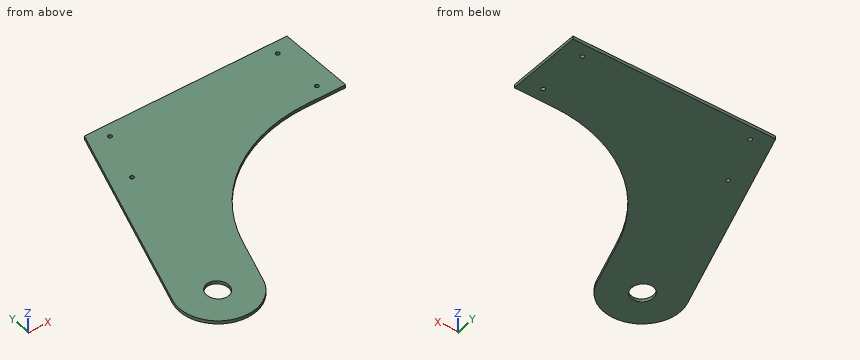
Autodesk Inventor part; units mm, degrees
ref_plane "YZ Plane" through (0, 0, 0) normal (1, 0, 0) x (0, 1, 0)
ref_plane "XZ Plane" through (0, 0, 0) normal (0, 1, 0) x (-1, 0, 0)
ref_plane "XY Plane" through (0, 0, 0) normal (0, 0, 1) x (1, 0, 0)
sketch "Sketch1" plane through (0, 0, 0) normal (0, 0, 1) x (1, 0, 0)
  arc A0 (219.754, -304.8) -> (225.7704, -296.4188) centre (219.754, -298.45) ccw
  line L0 (225.7704, -296.4188) -> (30.0819, 283.206)
  arc A1 (30.0819, 283.206) -> (-30.0819, 283.206) centre (0, 273.05) ccw
  line L1 (-30.0819, 283.206) -> (-225.7704, -296.4188)
  arc A2 (-225.7704, -296.4188) -> (-219.754, -304.8) centre (-219.754, -298.45) ccw
  line L2 (-219.754, -304.8) -> (219.754, -304.8)
  line L3 (-38.1, -17.4222) -> (-38.1, -222.25)
  arc A3 (-44.45, -228.6) -> (-38.1, -222.25) centre (-44.45, -222.25) ccw
  line L4 (-44.45, -228.6) -> (-113.6024, -228.6)
  arc A4 (-119.6188, -220.2188) -> (-113.6024, -228.6) centre (-113.6024, -222.25) ccw
  line L5 (-119.6188, -220.2188) -> (-50.4664, -15.391)
  arc A5 (-38.1, -17.4222) -> (-50.4664, -15.391) centre (-44.45, -17.4222) ccw
  line L6 (113.6024, -228.6) -> (44.45, -228.6)
  arc A6 (38.1, -222.25) -> (44.45, -228.6) centre (44.45, -222.25) ccw
  line L7 (38.1, -222.25) -> (38.1, -17.4222)
  arc A7 (50.4664, -15.391) -> (38.1, -17.4222) centre (44.45, -17.4222) ccw
  line L8 (50.4664, -15.391) -> (119.6188, -220.2188)
  arc A8 (113.6024, -228.6) -> (119.6188, -220.2188) centre (113.6024, -222.25) ccw
  circle A9 centre (-204.2059, -292.1) radius 2
  circle A10 centre (-187.0552, -241.3) radius 2
  circle A11 centre (187.0552, -241.3) radius 2
  circle A12 centre (204.2059, -292.1) radius 2
  circle A13 centre (19.05, -241.3) radius 2
  circle A14 centre (19.05, -292.1) radius 2
  circle A15 centre (-19.05, -292.1) radius 2
  circle A16 centre (-19.05, -241.3) radius 2
  circle A17 centre (8.89, 288.4479) radius 2
  circle A18 centre (-8.89, 288.4479) radius 2
  circle A19 centre (-17.78, 273.05) radius 2
  circle A20 centre (-8.89, 257.6521) radius 2
  circle A21 centre (8.89, 257.6521) radius 2
  circle A22 centre (17.78, 273.05) radius 2
  line L9 (0, -228.6) -> (-202.8739, -228.6)
  line L10 (0, -228.6) -> (0, -304.8)
  line L11 (-119.6188, -220.2188) -> (-208.2019, -482.6)
  line L12 (-225.7704, -296.4188) -> (-288.6275, -482.6)
  line L13 (-288.6275, -482.6) -> (-208.2019, -482.6)
  circle A23 centre (-235.5517, -444.5) radius 38.1
  circle A24 centre (-235.5517, -444.5) radius 10.668
  ellipse E0 centre (0, 273.05) end of major axis (-12.7, 273.05) minor radius 12.2673
  point P0 (0, 0)
  point P1 (-271.6499, -432.3128)
  point P2 (-199.4535, -456.6872)
  point P3 (-148.1744, -304.8)
  dimension "d0" = 21.336
  dimension "d1" = 254
extrude "Extrusion1" add sketch "Sketch1" along normal blind 3.175 contours L2 L11 L9 L4 L10 | L11 A23 L12 A2 L2 | L2 A2 L1 L9 L11 | A23
fillet "Fillet1" radius 152.4 1 edges at (-148.1744, -304.8, 1.5875)
ref_plane "Work Plane1" through (-235.5517, -444.5, 3.175) normal (0, -0.258819, 0.9659258) x (-1, 0, 0)
sketch "Sketch2" plane through (-235.5517, -444.5, 3.175) normal (0, -0.258819, 0.9659258) x (-1, 0, 0)
  ellipse E0 centre (0, 0) end of major axis (10.668, 0) minor radius 10.3045
  circle A0 centre (0, 0) radius 10.668
  point P0 (-235.5517, -428.5323)
  dimension "d6" = 21.336
sketch "Sketch3" plane through (0, 0, 3.175) normal (0, 0, 1) x (1, 0, 0)
  point P0 (0, 0)
extrude "Extrusion2" cut sketch "Sketch2" along normal through all both and the other way through all
sketch "Sketch4" plane through (0, 0, 3.175) normal (0, 0, 1) x (1, 0, 0)
  ellipse E0 centre (-235.5517, -444.5) end of major axis (-235.5517, -455.5443) minor radius 10.668 (-224.8837, -444.5) -> (-246.2197, -444.5) ccw
  ellipse E1 centre (-235.5517, -444.5) end of major axis (-235.5517, -455.5443) minor radius 10.668 (-246.2197, -444.5) -> (-224.8837, -444.5) ccw
  line L0 (-202.8739, -228.6) -> (-271.6499, -432.3128)
  arc A0 (-271.6499, -432.3128) -> (-199.4535, -456.6872) centre (-235.5517, -444.5) ccw
  arc A1 (-38.7755, -304.8) -> (-183.1684, -408.4512) centre (-38.7755, -457.2) ccw
  line L1 (-38.7755, -304.8) -> (0, -304.8)
  line L2 (0, -304.8) -> (0, -228.6)
  line L3 (0, -228.6) -> (-202.8739, -228.6)
  circle A2 centre (-19.05, -241.3) radius 2
  circle A3 centre (-19.05, -292.1) radius 2
  circle A4 centre (-204.2059, -292.1) radius 2
  circle A5 centre (-187.0552, -241.3) radius 2
  circle A6 centre (-187.0552, -241.3) radius 2
  circle A7 centre (-204.2059, -292.1) radius 2
  ellipse E2 centre (-235.5517, -443.6493) end of major axis (-235.5517, -454.6936) minor radius 10.668 (-224.8919, -444.082) -> (-246.2115, -444.082) ccw
  arc A8 (-246.2115, -444.082) -> (-224.8919, -444.082) centre (-235.5517, -444.5) ccw
  circle A9 centre (-19.05, -292.1) radius 2
  circle A10 centre (-19.05, -241.3) radius 2
  line L4 (-202.8739, -228.6) -> (-271.6499, -432.3128)
  line L5 (0, -228.6) -> (-202.8739, -228.6)
  line L6 (0, -304.8) -> (0, -228.6)
  line L7 (-38.7755, -304.8) -> (0, -304.8)
  arc A11 (-38.7755, -304.8) -> (-183.1684, -408.4512) centre (-38.7755, -457.2) ccw
  arc A12 (-271.6499, -432.3128) -> (-199.4535, -456.6872) centre (-235.5517, -444.5) ccw
  line L8 (-199.4535, -456.6872) -> (-183.1684, -408.4512)
  line L9 (-199.4535, -456.6872) -> (-183.1684, -408.4512)
  point P0 (0, 0)
extrude "Extrusion3" cut sketch "Sketch4" against normal through all contours A8 E0 | E0 E2
properties part number "FrameLeg" material "MDF Medium Density Fiberboard"
Input: part model. Units: mm. Frame: model coordinates. Coordinates: 2 decimals unless noted, no trailing zeros. Write each loop counter-clockwise with the first axis right and the second up, starting at its lowest first coordinate (ties: lowest second). Pieces come first, ordered by that corner, then holes. Notation, with made-up numbers: M 55,-2 L 89,-2 A18 cw 89,12 Z; hole C -28,-14.75 d2. An arc over 180 degrees is marked long. Answer as a JSON object with one key per item and string values. Group by question number.
(1) Contact query for flat-ended pins moving along their axis: P1, Ø1.5, axis at y = -380.5, z = 1, coming from the +X side; P2, Ø2.5, axis at x = -19.05, y = -241.3, coming from the -Z side; P3, Ø1.5, axis at x = -133.5, y = -323.5, coming from the -Z side. Output: stop coordinate, or through.
(2) Section B-B on y = -360. Output: boundary loops of the cut face in (x, z) (3 decimals), plus the area to 3 significant figures.
(3) Section C-C on x = -212. Output: boundary loops of the cut face in (y, z) (3 decimals).
(4) Section A-A on z = 2.3. Give the number of separate pieces and of enclosed holes in the cut face, plus the area to 3 significant figures.
(5) Ray query, line 1 along Y through (x, z) = (-19.05, 2.2); line 2 along X through (y, z) = (-292.1, 1.6); line 3 along X through (y, z) = (-241.3, 1). Return the intervals inside material, ascending. Write a range as [from, to].
Result set:
{
 "1": {"P1": "stops at x = -170.03", "P2": "passes through", "P3": "stops at z = 0"},
 "2": {"outline": "M -247.236,0 L -156.155,0 L -156.155,3.175 L -247.236,3.175 Z", "area": "289 mm2"},
 "3": {"outline": "M -474.449,0 L -255.631,0 L -255.631,3.175 L -474.449,3.175 Z"},
 "4": {"separate pieces": "1", "enclosed holes": "5", "area": "31,700 mm2"},
 "5": {"line 1": "y = [-304.8, -294.1], [-290.1, -243.3], [-239.3, -228.6]", "line 2": "x = [-224.31, -206.21], [-202.21, -21.05], [-17.05, 0]", "line 3": "x = [-207.16, -189.06], [-185.06, -21.05], [-17.05, 0]"}
}
